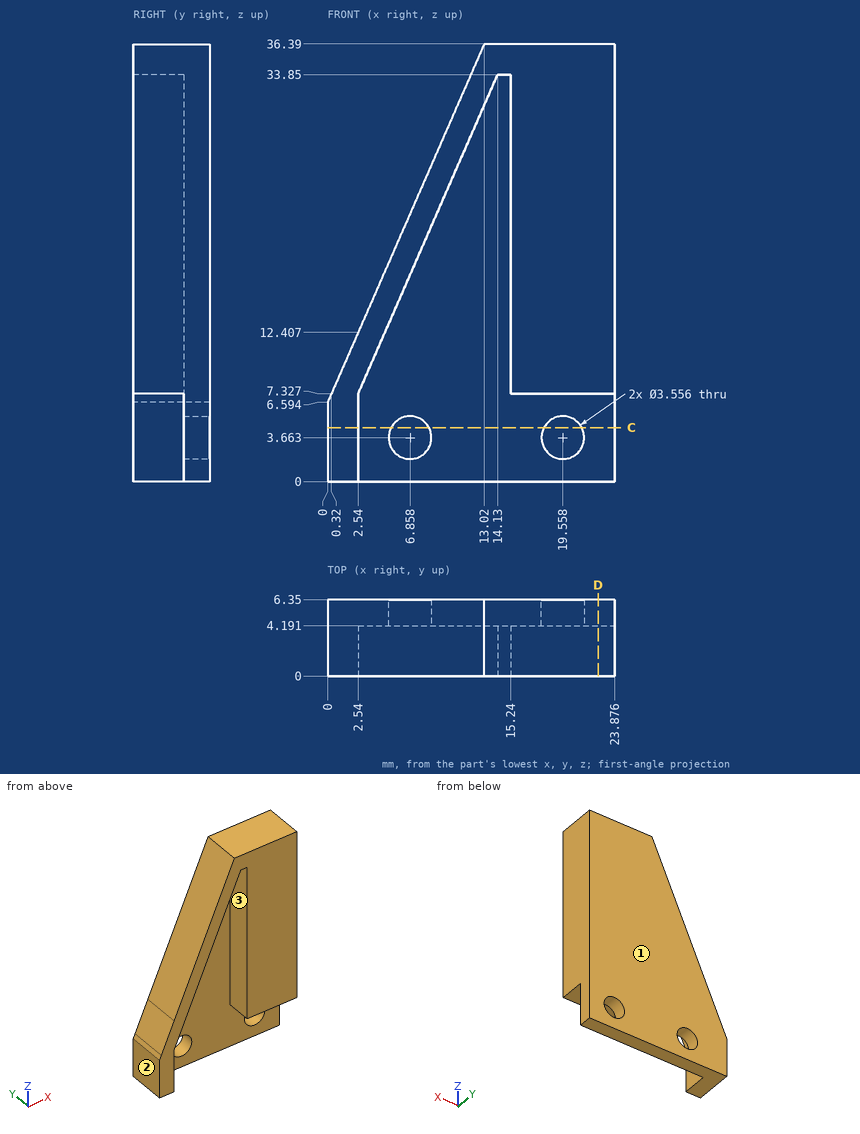
Verification items for this drawing (mm, ordinates from the low corner). Give positions to 0.01 mm unless a question says otherwise; leave off trailing zeros. Write each loop counter-clockwise with the first axis right and the second up, starting at its lowest first coordinate (ties: lowest second). Pieces come first, ordered by that corner, then holes. Notation, with made-up numbers: (81.25, -10) -> (101.25, -10) arc R20 ccw to (101.25, 27) -> close; hole circle Ø7 at (-28, -6). An arc over 180 degrees is marked (long way). Write item = value, one per line.
Item 1: Release check for a two-part mould opening along X. For the marked faces 1, 2 and 3 record: +X half, -X half, draft (parallel to the pull), parting line (faces both ways), or undercut.
Output:
face_1 = draft
face_2 = -X half
face_3 = undercut
Item 2: Scan lines: probe 1 along Y at (x, z) = (10.25, 10); probe 2 along X at (y, z) = (3.75, 2); probe 3 along X at (y, z) = (4, 20.5) (1 decimal). Record each from-to range of solid material in increasing order. Write a range as from..to.
Output:
probe_1 = 4.19..6.35
probe_2 = 0..2.54
probe_3 = 6.1..8.3, 15.2..23.9
Item 3: Sectioned sample at C-C on z = 4.5. Record the boundary of the cut face in (x, y).
Output:
outline = (0, 0) -> (2.54, 0) -> (2.54, 4.19) -> (5.29, 4.19) -> (5.29, 6.35) -> (0, 6.35) -> close; (8.43, 4.19) -> (17.99, 4.19) -> (17.99, 6.35) -> (8.43, 6.35) -> close; (21.13, 4.19) -> (23.88, 4.19) -> (23.88, 6.35) -> (21.13, 6.35) -> close
Item 4: Gauge pin test, flat ends, axial feed: pin 1 (0.6 mm diameter, centred on x = 15, y = 2, fed in from -Z); pin 2 (2 mm diameter, centred on y = 1.5, z = 26.5, fed in from -X); pin 3 (1.3 mm diameter, centred on y = 2.5, z = 5.5, fed in from +X); pin 4 (10.5 mm diameter, centred on x = 17.5, z = 18.5, fed in from -Y). Record the tip position at first contact, or that the pin passes through.
Output:
pin_1 = 7.33
pin_2 = 8.26
pin_3 = 2.54
pin_4 = 0
Item 5: Sectioned sample at D-D on x = 22.5. Record the boundary of the cut face in (y, z), and give its area (3 significant figures).
Output:
outline = (0, 7.33) -> (4.19, 7.33) -> (4.19, 0) -> (6.35, 0) -> (6.35, 36.39) -> (0, 36.39) -> close
area = 200 mm^2
